from build123d import *

# Parameters (mm, degrees)
BOSS_EXTRUDE1_DEPTH = 12.7


with BuildPart() as part:
    # Sketch1 → Boss-Extrude1 (new body)
    with BuildSketch(Plane(origin=(0, 0, 0), x_dir=(0, 0, -1), z_dir=(1, 0, 0))):
        Polygon((0, 0), (12.7, 0), (12.7, -12.7), (25.4, -12.7), (25.4, 0), (38.1, 0), (38.1, -12.7), (50.8, -12.7), (50.8, 0), (63.5, 0), (63.5, -12.7), (76.2, -12.7), (76.2, 0), (88.9, 0), (88.9, -12.7), (101.6, -12.7), (101.6, 0), (114.3, 0), (114.3, 12.7), (101.6, 12.7), (101.6, 25.4), (114.3, 25.4), (114.3, 38.1), (101.6, 38.1), (101.6, 50.8), (114.3, 50.8), (114.3, 63.5), (101.6, 63.5), (0, 63.5), align=None)
    extrude(amount=BOSS_EXTRUDE1_DEPTH)


solid = part.part
CAD build for the part. Positions are in the model's coordinates, mm. A direction names the side the tool comes from. Round coordinates to 2 decimals unless told otherwise and drop trailing zeros. Order: outer loops, then holes, each group sorted by start corner. A loop starts at its lowest first (then second) coordinate and runs counter-clockwise, first axis right, second up. Notation, with made-up numbers: (53.5, 68.5) - (68.5, 68.5) arc R9 cw to (68.5, 79.5) - close; hole circle Ø5 at (-26.75, -35.5). An arc over 180 degrees is marked (long way). Return JSON: item names as keys, results as strings.
(1) Cut at C-C (z = -59.5). Give the cut face in (x, y).
Answer key:
{"outline": "(0, 0) - (12.7, 0) - (12.7, 63.5) - (0, 63.5) - close"}
(2) Wall check: probe 1 along Z at (x, y) = (2.75, -2); probe 2 along Y at (x, z) = (7.25, -80.5); probe 3 along Z at (x, y) = (9.5, 49). Give the ranges that are in metal, low to high. Write a range as from..to.
Answer key:
{"probe 1": "z = -101.6..-88.9, -76.2..-63.5, -50.8..-38.1, -25.4..-12.7", "probe 2": "y = 0..63.5", "probe 3": "z = -101.6..0"}
(3) Cut at D-D (y = 18). Give the cut face in (x, z).
Answer key:
{"outline": "(0, -101.6) - (12.7, -101.6) - (12.7, 0) - (0, 0) - close"}
(4) Tool access for faces 5 (the face through (6, 38.1, -108)), 6 (the face through (6, 0, -108)), 7 (the face through (6, -6, -50.8)): list every direction of +Z, -Z, +X, -X, +Y, -Y with a clear straight run to the whole face (end or side of a thin tool).
Answer key:
{"face 5": "-Z, +X, -X", "face 6": "-Z, +X, -X, -Y", "face 7": "+X, -X, -Y"}
(5) Pull direction Z, two halves, no side cores. Call faces 1 (the face through (6, 32, -114.3)), 2 (the face through (6, -6, -63.5)), 3 (the face through (6, 0, -82)), 4 (the face through (6, -12.7, -44)): +Z half, -Z half, draft (parallel to the pull), parting line (faces both ways), or undercut.
Answer key:
{"face 1": "-Z half", "face 2": "undercut", "face 3": "undercut", "face 4": "draft"}
(6) Cut at B-B (x = 7). Give the cut face in (y, z).
Answer key:
{"outline": "(-12.7, -101.6) - (0, -101.6) - (0, -114.3) - (12.7, -114.3) - (12.7, -101.6) - (25.4, -101.6) - (25.4, -114.3) - (38.1, -114.3) - (38.1, -101.6) - (50.8, -101.6) - (50.8, -114.3) - (63.5, -114.3) - (63.5, 0) - (0, 0) - (0, -12.7) - (-12.7, -12.7) - (-12.7, -25.4) - (0, -25.4) - (0, -38.1) - (-12.7, -38.1) - (-12.7, -50.8) - (0, -50.8) - (0, -63.5) - (-12.7, -63.5) - (-12.7, -76.2) - (0, -76.2) - (0, -88.9) - (-12.7, -88.9) - close"}
(7) Pin check, flat tips, straight feed: pin 1 Ø4 at (x, y) = (6.5, -5) entering from -Z; pin 2 Ø4 at (x, z) = (7, -79.5) entering from -Y. Stop position of each tip, or through.
Answer key:
{"pin 1": "stops at z = -101.6", "pin 2": "stops at y = 0"}
(8) Cut at A-A (y = -3.5). Give the cut face in (x, z).
Answer key:
{"outline": "(0, -101.6) - (12.7, -101.6) - (12.7, -88.9) - (0, -88.9) - close; (0, -76.2) - (12.7, -76.2) - (12.7, -63.5) - (0, -63.5) - close; (0, -50.8) - (12.7, -50.8) - (12.7, -38.1) - (0, -38.1) - close; (0, -25.4) - (12.7, -25.4) - (12.7, -12.7) - (0, -12.7) - close"}
